Input: dimensioned drawing with shaded views. Units: mm. Origin: part minimum x, y, z. A direction names the side the tool comes from. Coordinates: 2 decimals unless noted, no trailing zeros. Loops run counter-clockwise (first coordinate to the right, second up) from the corner with the lowest first, then second, coordinate; pieces in that order, holes last.
Item 1: Ray query, line 1 along Z through (x, y) = (130, 5.5); line 2 along X through (y, z) = (18.5, 43). Return the intervals inside material, ascending.
Item 2: Section C-C on z = 47. Return loops of the section in (x, y), and give its area (3 significant figures).
Item 3: Pull-direction query (X, two-part tool) for the marked faces 1, 2 and 3; classes: released by +X, released by -X, zero draft, split by the parting line, or undercut.
Item 4: Section A-A on x = 72.5. Return loops of the section in (y, z), and give its area (3 significant figures).
Item 5: Reachability of the marked faces 4 and 5 from +Z, -Z, +X, -X, +Y, -Y: full face, straight path, thin tool, end or side. Return the list, or none.
Item 6: Section B-B on y = 7. Return loops of the section in (x, z), and give its area (3 significant figures).
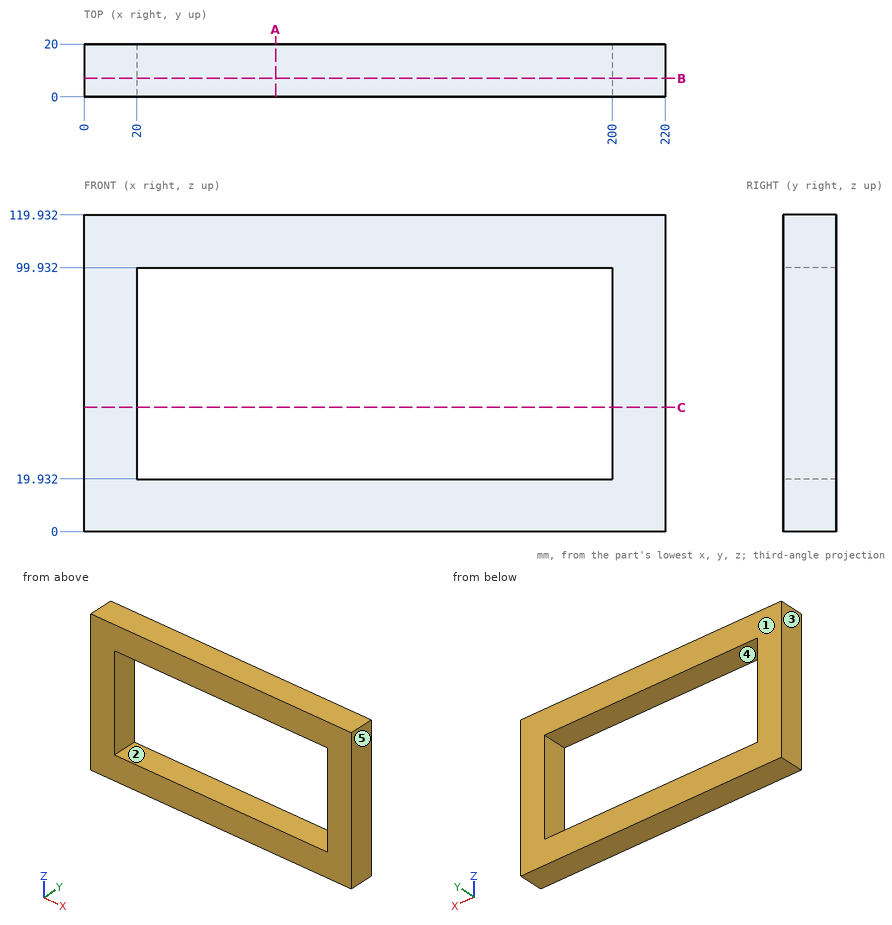
Results found:
1. line 1: z = 0 to 19.93, 99.93 to 119.93
1. line 2: x = 0 to 20, 200 to 220
2. outline: (0, 0) - (20, 0) - (20, 20) - (0, 20) - close; (200, 0) - (220, 0) - (220, 20) - (200, 20) - close
2. area: 800 mm2
3. face 1: zero draft
3. face 2: undercut
3. face 3: released by -X
4. outline: (0, 0) - (20, 0) - (20, 19.93) - (0, 19.93) - close; (0, 99.93) - (20, 99.93) - (20, 119.93) - (0, 119.93) - close
4. area: 799 mm2
5. face 4: +Y, -Y
5. face 5: +Z, -Z, +X, +Y, -Y
6. outline: (0, 0) - (220, 0) - (220, 119.93) - (0, 119.93) - close; hole (20, 19.93) - (200, 19.93) - (200, 99.93) - (20, 99.93) - close
6. area: 12,000 mm2
